Check sheet for the modelled part. Datum: model origin and axes. Units: mm. A direction names the side the tool comes from. Coordinates: 2 decimals unless noted, no trailing zeros. Loops run counter-clockwise (first coordinate to the right, second up) from the corner with the lowest first, then second, coordinate; pieces in that order, holes last.
from build123d import *

# Parameters (mm, degrees)
SKETCH1_R           = 1.125
SKETCH1_R_2         = 1.54
BOSS_EXTRUDE1_DEPTH = 13
SKETCH2_R           = 1.125
CUT_EXTRUDE1_DEPTH  = 3
CUT_EXTRUDE1_TAPER  = -10
FILLET1_R           = 1
FILLET2_R           = 1
FILLET3_R           = 1
FILLET4_R           = 1


with BuildPart() as part:
    # Sketch1 → Boss-Extrude1 (new, symmetric)
    with BuildSketch(Plane.XY):
        with BuildLine():
            Line((8, 5.57), (8, 0))
            ThreePointArc((8, 0), (7.692956073, -2.195091538), (6.795393285, -4.221685695))
            Line((6.795393285, -4.221685695), (3.618574799, -9.335219142))
            ThreePointArc((3.618574799, -9.335219142), (-9.482620111, -9.856988447), (-5.1153336, 2.505873673))
            Line((-5.1153336, 2.505873673), (-2.830230063, 3.104309401))
            ThreePointArc((-2.830230063, 3.104309401), (-1.020355645, 4.136406118), (0.029802368, 5.93586081))
            ThreePointArc((0.029802368, 5.93586081), (2.498115044, 10.172124839), (7.138397607, 8.589001937))
            ThreePointArc((7.138397607, 8.589001937), (7.780383364, 7.13977159), (8, 5.57))
        make_face()
        with Locations(Location((3.85133489, 6.546425452, 0), (0, 0, 180))):
            Circle(SKETCH1_R, mode=Mode.SUBTRACT)
        with Locations(Location((-3.108864553, -5.155750304, 0), (0, 0, 180))):
            Circle(SKETCH1_R_2, mode=Mode.SUBTRACT)
    extrude(amount=BOSS_EXTRUDE1_DEPTH, both=True)

    # Sketch2 → Cut-Extrude1 (cut)
    with BuildSketch(Plane.XY.offset(13)):
        with BuildLine():
            Line((8, 0.172124839), (8, 5.57))
            ThreePointArc((8, 5.57), (7.780383364, 7.13977159), (7.138397607, 8.589001937))
            ThreePointArc((7.138397607, 8.589001937), (2.498115044, 10.172124839), (0.029802368, 5.93586081))
            ThreePointArc((0.029802368, 5.93586081), (-1.020355645, 4.136406118), (-2.830230063, 3.104309401))
            Line((-2.830230063, 3.104309401), (-3.781962396, 2.855064401))
            Line((-3.781962396, 2.855064401), (8, 0.172124839))
        make_face()
        with Locations(Location((3.85133489, 6.546425452, 0), (0, 0, 180))):
            Circle(SKETCH2_R, mode=Mode.SUBTRACT)
    cut_extrude1 = extrude(amount=-CUT_EXTRUDE1_DEPTH, taper=CUT_EXTRUDE1_TAPER, mode=Mode.SUBTRACT)

    # Mirror1: Cut-Extrude1 across plane
    add(cut_extrude1.mirror(Plane.XY), mode=Mode.SUBTRACT)

    # Fillet1
    fillet1_edges = [part.edges().sort_by_distance(p)[0] for p in [
        (2.109018802, 1.51359462, -13),
    ]]
    fillet(fillet1_edges, radius=FILLET1_R)

    # Fillet2
    fillet2_edges = [part.edges().sort_by_distance(p)[0] for p in [
        (2.109018802, 1.51359462, 13),
    ]]
    fillet(fillet2_edges, radius=FILLET2_R)

    # Fillet3
    fillet3_edges = [part.edges().sort_by_distance(p)[0] for p in [
        (1.550728698, 1.09820349, -10),
    ]]
    fillet(fillet3_edges, radius=FILLET3_R)

    # Fillet4
    fillet4_edges = [part.edges().sort_by_distance(p)[0] for p in [
        (1.550728698, 1.09820349, 10),
    ]]
    fillet(fillet4_edges, radius=FILLET4_R)


solid = part.part
(1) Set-up check for faces 1 (the face through (4, 5, 10)), 2 (the face through (4, 5, -10)), 3 (the face through (5.23, -6.74, 0.18)): record each of +Z, -Z, +X, -X, +Y, -Y from which the full face is reachable in a straight line by a thin tool's end or side.
(2) Section check D-D, the plane y = -9. Enter the section's corners in (x, z), plus the area to 3 significant figures.
(3) Draft check along Y on faces 4 (the face through (2.812, 6.977, -0.14)), 5 (the face through (-4, 2.8, 0.2)), 6 (the face through (-2.78, -3.65, -0.18)), 7 (the face through (7.7, -2.17, 0.18)). Enter one of: pulls with the +Y half, pulls with the -Y half, needs draft (parallel to the pull), parting line crosses it, or undercut.
(4) Section check B-B, the plane z = -8.25. Enter the section's corners in (x, y) (3 decimals).
(5) Section check A-A, the plane y = -6. Enter the section's corners in (x, z).
(6) Scan lines: line 1 along Z through (x, y) = (0.5, 7.25); line 2 along X through (y, z) = (6.25, 4.25); line 3 along Z through (x, y) = (-5, 2). Record each from-to range of solid material in increasing order.
(7) Gauge pin test, flat ends, axial feed: P1, Ø1, axis at x = 1, z = -9, coming from the +Y side; P2, Ø1.5, axis at x = -3.5, y = 5, coming from the +Z side; P3, Ø3.5, axis at x = 3.85, y = 6.55, coming from the +Z side; P4, Ø1, axis at x = -4, y = 2.5, coming from the +Z side. Record the tip position at first contact, or that the pin passes through.
(8) Section check C-C, the plane x = -6.5. Enter the section's corners in (y, z), plus the area to 3 significant figures.
Determined:
1. face 1: +Z, +X, +Y
1. face 2: -Z, +X, +Y
1. face 3: +Z, -Z, +X, -Y
2. outline: (-10.03, -13) - (3.83, -13) - (3.83, 13) - (-10.03, 13) - close
2. area: 360 mm2
3. face 4: undercut
3. face 5: pulls with the +Y half
3. face 6: undercut
3. face 7: pulls with the -Y half
4. outline: (-5.115, 2.506) arc R7.92 ccw (long way) to (3.619, -9.335) - (6.795, -4.222) arc R8 ccw to (8, 0) - (8, 5.57) arc R5.72 ccw to (7.138, 8.589) arc R3.87 ccw to (0.03, 5.936) arc R4.02 cw to (-2.83, 3.104) - close; hole circle Ø3.08 at (-3.109, -5.156); hole circle Ø2.25 at (3.851, 6.546)
5. outline: (-10.98, -13) - (-4.4, -13) - (-4.4, 13) - (-10.98, 13) - close; (-1.82, -13) - (5.69, -13) - (5.69, 13) - (-1.82, 13) - close
6. line 1: z = -10 to 10
6. line 2: x = -0.01 to 2.77, 4.94 to 7.96
6. line 3: z = -13 to 13
7. P1: stops at y = 9.62
7. P2: passes through
7. P3: stops at z = 10
7. P4: stops at z = 12.95
8. outline: (-12.31, -13) - (2, -13) - (2, 13) - (-12.31, 13) - close
8. area: 372 mm2
